Autodesk Inventor part; units mm, degrees
ref_plane "YZ Plane" through (0, 0, 0) normal (1, 0, 0) x (0, 1, 0)
ref_plane "XZ Plane" through (0, 0, 0) normal (0, 1, 0) x (-1, 0, 0)
ref_plane "XY Plane" through (0, 0, 0) normal (0, 0, 1) x (1, 0, 0)
sketch "Sketch2" plane through (0, 0, 0) normal (0, 1, 0) x (-1, 0, 0)
  line L0 (0, 0) -> (-170, 0)
  line L1 (-170, 0) -> (-170, -160)
  line L2 (-170, -160) -> (0, -160)
  line L3 (0, -160) -> (0, 0)
  line L4 (-8, -8) -> (-162, -8)
  line L5 (-162, -8) -> (-162, -152)
  line L6 (-162, -152) -> (-8, -152)
  line L7 (-8, -152) -> (-8, -8)
  dimension "d0" = 170
  dimension "d1" = 160
  dimension "d2" = 154
  dimension "d3" = 144
  dimension "d4" = 8
  dimension "d5" = 8
extrude "Extrusion1" add sketch "Sketch2" along normal blind 15
extrude "Extrusion2" add sketch "Sketch2" along normal blind 3 contours L7 L6 L5 L4
sketch "Sketch3" plane through (0, 0, 0) normal (0, 0, 1) x (1, 0, 0)
  line L0 (0, 0) -> (0, 7.5)
  line L1 (0, 0) -> (0, 15)
  line L2 (0, 7.5) -> (170, 7.5)
  line L3 (170, 0) -> (170, 15)
  line L4 (0, 7.5) -> (40, 7.5)
  line L5 (170, 7.5) -> (130, 7.5)
  dimension "d10" = 40
  dimension "d11" = 40
hole "Hole1" at (130, 7.5, 0) direction (0, 0, -1) diameter 6 depth 160
properties part number "baseplate"
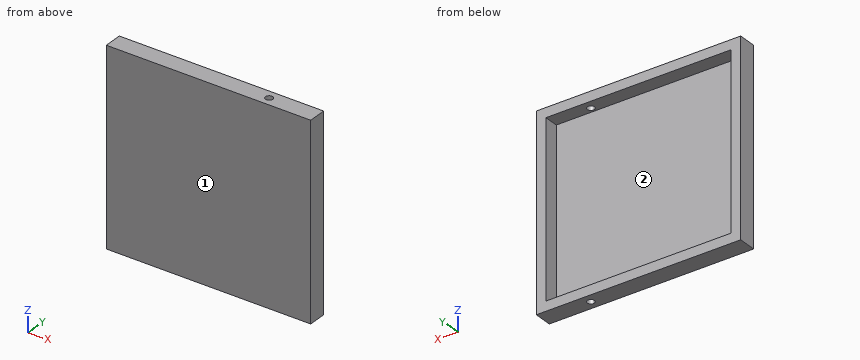
Part model, mm, in its own coordinate system. Face numbers are marked on the shaded views. Round coordinates to 2 decimals unless told otherwise and drop trailing zeros. Order: outer loops, then holes, each group sorted by start corner. A loop starts at its lowest first (then second) coordinate and runs counter-clockwise, first axis right, second up. Notation, with made-up numbers: (-12, -35) -> (0, -35) arc R21 cw to (0, -13) -> close; hole circle Ø10 at (-21.75, -25.5). An arc over 180 degrees is marked (long way). Put each result on its own line as item: value.
Q1. Band-saw the part on A-A (x = 130). Give the cut face in (y, z), and give its area (3 significant figures).
From the geometry:
outline: (0, -160) -> (4.5, -160) -> (4.5, -152) -> (3, -152) -> (3, -8) -> (4.5, -8) -> (4.5, 0) -> (0, 0) -> close; (10.5, -160) -> (15, -160) -> (15, -152) -> (10.5, -152) -> close; (10.5, -8) -> (15, -8) -> (15, 0) -> (10.5, 0) -> close
area: 576 mm2
Q2. Pull direction Z, two halves, no side cores. Call the marked faces 1 and 2: pulls with the +Z half, pulls with the -Z half, needs draft (parallel to the pull), parting line crosses it, or undercut.
From the geometry:
face 1: needs draft
face 2: undercut
Q3. Wall check: line 1 (X direction, y = 7.5, z = -2); line 2 (X direction, y = 5, z = -15); line 3 (Z direction, x = 13, y = 3.5). Give the ranges that are in metal, low to high. Write a range as [from, to].
From the geometry:
line 1: x = [0, 127], [133, 170]
line 2: x = [0, 8], [162, 170]
line 3: z = [-160, -152], [-8, 0]
Q4. Pin check, flat tips, straight feed: pin 1 Ø1.5 at (x, z) = (141, -88.5) entering from +Y; pin 2 Ø3.5 at (x, y) = (130, 7.5) entering from -Z. Stop position of each tip, or through.
From the geometry:
pin 1: stops at y = 3
pin 2: passes through
Q5. Band-saw the part on D-D (x = 46.5). Give the cut face in (y, z).
From the geometry:
outline: (0, -160) -> (15, -160) -> (15, -152) -> (3, -152) -> (3, -8) -> (15, -8) -> (15, 0) -> (0, 0) -> close
Q6. Band-saw the part on B-B (y = 7.5). Give the cut face in (x, z).
From the geometry:
outline: (0, -160) -> (127, -160) -> (127, -152) -> (8, -152) -> (8, -8) -> (127, -8) -> (127, 0) -> (0, 0) -> close; (133, -160) -> (170, -160) -> (170, 0) -> (133, 0) -> (133, -8) -> (162, -8) -> (162, -152) -> (133, -152) -> close
Q7. Band-saw the part on C-C (z = -98). Give the cut face in (x, y).
From the geometry:
outline: (0, 0) -> (170, 0) -> (170, 15) -> (162, 15) -> (162, 3) -> (8, 3) -> (8, 15) -> (0, 15) -> close
